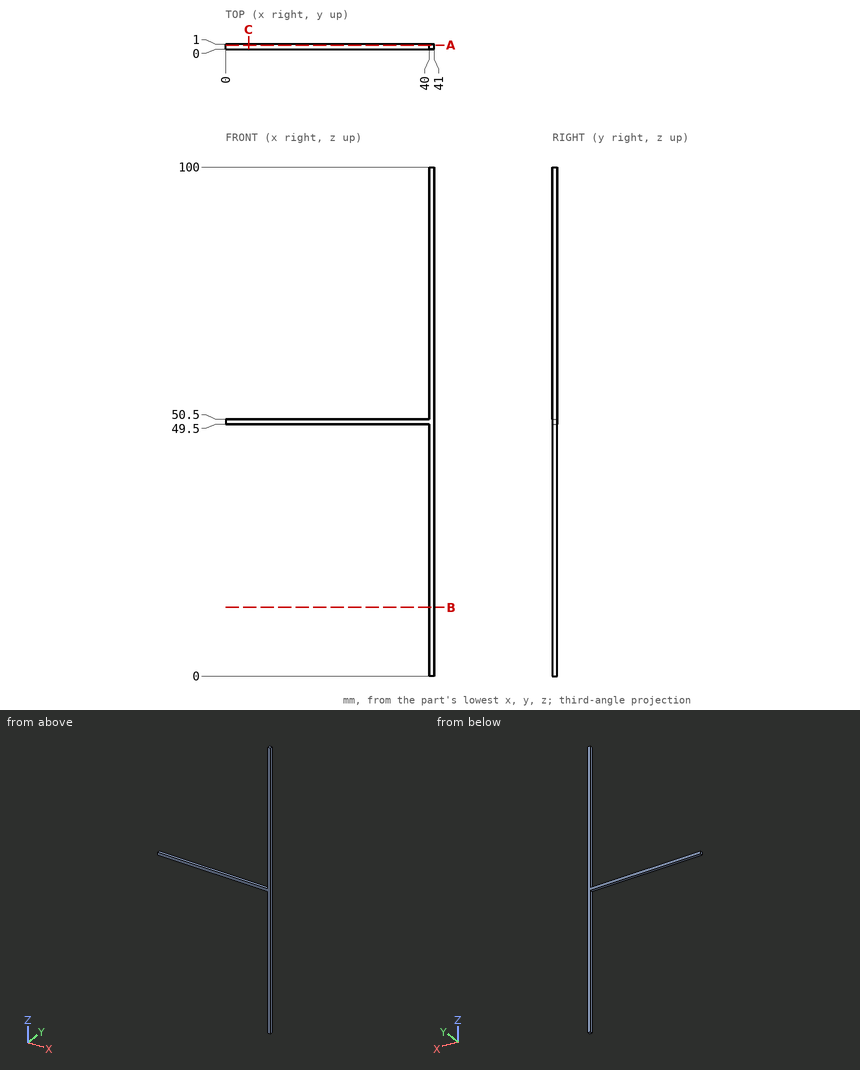
Geometry: see drawing. Coordinates: mm, zero at the bounding-box minimum. Coordinates: 2 decimals unless noted, no trailing zeros. Loops run counter-clockwise (first coordinate to the right, second up) from the corner with the lowest first, then second, coordinate; pieces in that order, holes last. Notation, with made-up numbers: (16.25, 29) - (26.25, 29) arc R18 cw to (26.25, 53) - close; hole circle Ø4 at (-28.75, -10). An arc over 180 degrees is marked (long way). Answer in a Markdown table with one row per item.
(1) Cut plane C-C on x = 4.5. Output: boundary loops of the cut face in (y, z), plus the area to 3 significant figures.
Model answer:
| item | result |
|---|---|
| outline | (0, 49.5) - (1, 49.5) - (1, 50.5) - (0, 50.5) - close |
| area | 1.00 mm² |
(2) Cut plane B-B on z = 13.5. Output: boundary loops of the cut face in (x, y).
Model answer:
| item | result |
|---|---|
| outline | (40, 0) - (41, 0) - (41, 1) - (40, 1) - close |
(3) Cut plane A-A on y = 0.8. Output: boundary loops of the cut face in (x, z), plus the area to 3 significant figures.
Model answer:
| item | result |
|---|---|
| outline | (0, 49.5) - (40, 49.5) - (40, 0) - (41, 0) - (41, 100) - (40, 100) - (40, 50.5) - (0, 50.5) - close |
| area | 140 mm² |
(4) Material intervals for L1, parallel to X at y = 0.4, z = 58.5; L2, parallel to Z at x = 22, y = 0.1, sorted ascending. Write a range as from..to.
Model answer:
| item | result |
|---|---|
| L1 | x = 40..41 |
| L2 | z = 49.5..50.5 |
